Work out the finished part from the listing and answer in its coordinate system (mm). A direction names the side the tool comes from. Coordinates: 2 decimals unless noted, no trailing zeros. Use a Markdown table: item, result.
from build123d import *

# Parameters (mm, degrees)
SKETCH_W        = 213
SKETCH_H        = 360
PAD_DEPTH       = 6.5
SKETCH001_R     = 5.2
POCKET_DEPTH    = 3.4
SKETCH002_R     = 3.2
POCKET001_DEPTH = 3.1


with BuildPart() as part:
    # Sketch → Pad (new body)
    with BuildSketch(Plane.XY):
        with Locations((106.5, 180)):
            Rectangle(SKETCH_W, SKETCH_H)
    extrude(amount=PAD_DEPTH)

    # Sketch001 (on Face6 of Pad) → Pocket (cut)
    with BuildSketch(Plane.XY.offset(6.5)):
        with Locations((106.5, 350)):
            Circle(SKETCH001_R)
        with Locations((16.5, 240)):
            Circle(SKETCH001_R)
        with Locations((16.5, 120)):
            Circle(SKETCH001_R)
        with Locations((196.5, 240)):
            Circle(SKETCH001_R)
        with Locations((196.5, 120)):
            Circle(SKETCH001_R)
        with Locations((106.5, 10)):
            Circle(SKETCH001_R)
    extrude(amount=-POCKET_DEPTH, mode=Mode.SUBTRACT)

    # Sketch002 (on Face17 of Pocket) → Pocket001 (cut)
    with BuildSketch(Plane.XY.offset(3.1)):
        with Locations((106.5, 350)):
            Circle(SKETCH002_R)
        with Locations((16.5, 240)):
            Circle(SKETCH002_R)
        with Locations((16.5, 120)):
            Circle(SKETCH002_R)
        with Locations((196.5, 240)):
            Circle(SKETCH002_R)
        with Locations((196.5, 120)):
            Circle(SKETCH002_R)
        with Locations((106.5, 10)):
            Circle(SKETCH002_R)
    extrude(amount=-POCKET001_DEPTH, mode=Mode.SUBTRACT)


solid = part.part
(1) Straight lines are drawn through the part: L1, parallel to Y at x = 16.5, z = 0.9; L2, parallel to Y at x = 16.5, z = 5.5; L3, parallel to X at y = 350, z = 1.8. For each, find the intervals that lie inside material, in ascending order.
Conclusion:
| item | result |
|---|---|
| L1 | 0 to 116.8, 123.2 to 236.8, 243.2 to 360 |
| L2 | 0 to 114.8, 125.2 to 234.8, 245.2 to 360 |
| L3 | 0 to 103.3, 109.7 to 213 |
(2) Given P1, Ø11.5, axis at x = 18.5, y = 118, coming from the +Z side; P2, Ø5, axis at x = 106.5, y = 10, coming from the -Z side; P3, Ø3, axis at x = 18.5, y = 242, coming from the +Z side, each flat-ended and moving along its own axis, determine where each tip first touches the part or whether it passes through.
Conclusion:
| item | result |
|---|---|
| P1 | z = 6.5 |
| P2 | through |
| P3 | z = 3.1 |
(3) Which of the six approach directions +Z, -Z, +X, -X, +Y, -Y give full straight-line access (tool end or side, diameter ignored) to faces 5 (the flat face through (110, 10, 3.1)), 6 (the cylindrical face through (15.806, 236.876, 1.572))?
Conclusion:
| item | result |
|---|---|
| face 5 | +Z |
| face 6 | +Z, -Z |
(4) Determine the mould class of faces 1 (the flat face through (105, 0, 3)), 2 (the cylindrical face through (192.667, 243.514, 4.824)), 3 (the flat face through (105, 360, 3)), 4 (the flat face through (105, 183, 0)) for opening direction Y: pulls with the +Y half, pulls with the -Y half, needs draft (parallel to the pull), parting line crosses it, or undercut.
Conclusion:
| item | result |
|---|---|
| face 1 | pulls with the -Y half |
| face 2 | undercut |
| face 3 | pulls with the +Y half |
| face 4 | needs draft |
